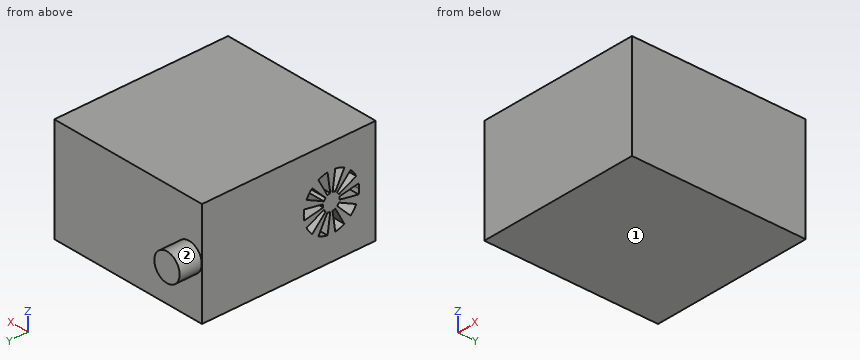
```python
from build123d import *

# Parameters (mm, degrees)
SKETCH1_W           = 73
SKETCH1_H           = 47
BOSS_EXTRUDE1_DEPTH = 78.5
SKETCH2_R           = 6.25
BOSS_EXTRUDE2_DEPTH = 10
CUT_EXTRUDE1_DEPTH  = 10


with BuildPart() as part:
    # Sketch1 → Boss-Extrude1 (new body)
    with BuildSketch(Plane(origin=(0, 0, 0), x_dir=(1, 0, 0), z_dir=(0, 1, 0))):
        with Locations((36.5, 23.5)):
            Rectangle(SKETCH1_W, SKETCH1_H)
    extrude(amount=BOSS_EXTRUDE1_DEPTH)

    # Sketch2 → Boss-Extrude2 (add)
    with BuildSketch(Plane(origin=(0, 78.5, 0), x_dir=(1, 0, 0), z_dir=(0, 1, 0))):
        with Locations(Location((6.35, 23.5, 0), (0, 0, 90))):
            Circle(SKETCH2_R)
    extrude(amount=BOSS_EXTRUDE2_DEPTH)

    # Sketch3 → Cut-Extrude1 (cut)
    with BuildSketch(Plane.ZY):
        with BuildLine():
            ThreePointArc((-21.329397779, 32.310096913), (-22.410553216, 32.452433726), (-23.5, 32.5))
            Line((-23.5, 32.5), (-23.5, 23.75))
            ThreePointArc((-23.5, 23.75), (-23.173165965, 23.735730118), (-22.848819334, 23.693029074))
            Line((-22.848819334, 23.693029074), (-21.329397779, 32.310096913))
        make_face()
        with BuildLine():
            Line((-23.5, 23.75), (-23.5, 32.5))
            ThreePointArc((-23.5, 32.5), (-24.589446784, 32.452433726), (-25.670602221, 32.310096913))
            Line((-25.670602221, 32.310096913), (-24.151180666, 23.693029074))
            ThreePointArc((-24.151180666, 23.693029074), (-23.826834035, 23.735730118), (-23.5, 23.75))
        make_face()
        with BuildLine():
            Line((-18.020360665, 31.234925579), (-21.8561082, 23.370477674))
            ThreePointArc((-21.8561082, 23.370477674), (-21.295805304, 23.033813729), (-20.802475749, 22.604968889))
            Line((-20.802475749, 22.604968889), (-14.508252496, 28.683229631))
            ThreePointArc((-14.508252496, 28.683229631), (-16.152684346, 30.11271243), (-18.020360665, 31.234925579))
        make_face()
        with BuildLine():
            Line((-12.463155089, 25.868394535), (-20.188946527, 21.76051836))
            ThreePointArc((-20.188946527, 21.76051836), (-19.933538064, 21.158813729), (-19.786494742, 20.521899129))
            Line((-19.786494742, 20.521899129), (-11.121649141, 21.739663762))
            ThreePointArc((-11.121649141, 21.739663762), (-11.611793546, 23.86271243), (-12.463155089, 25.868394535))
        make_face()
        with BuildLine():
            Line((-11.121649141, 18.260336238), (-19.786494742, 19.478100871))
            ThreePointArc((-19.786494742, 19.478100871), (-19.933538064, 18.841186271), (-20.188946527, 18.23948164))
            Line((-20.188946527, 18.23948164), (-12.463155089, 14.131605465))
            ThreePointArc((-12.463155089, 14.131605465), (-11.611793546, 16.13728757), (-11.121649141, 18.260336238))
        make_face()
        with BuildLine():
            Line((-21.8561082, 16.629522326), (-18.020360665, 8.765074421))
            ThreePointArc((-18.020360665, 8.765074421), (-16.152684346, 9.88728757), (-14.508252496, 11.316770369))
            Line((-14.508252496, 11.316770369), (-20.802475749, 17.395031111))
            ThreePointArc((-20.802475749, 17.395031111), (-21.295805304, 16.966186271), (-21.8561082, 16.629522326))
        make_face()
        with BuildLine():
            Line((-23.5, 16.25), (-23.5, 7.5))
            ThreePointArc((-23.5, 7.5), (-22.410553216, 7.547566274), (-21.329397779, 7.689903087))
            Line((-21.329397779, 7.689903087), (-22.848819334, 16.306970926))
            ThreePointArc((-22.848819334, 16.306970926), (-23.173165965, 16.264269882), (-23.5, 16.25))
        make_face()
        with BuildLine():
            ThreePointArc((-25.670602221, 7.689903087), (-24.589446784, 7.547566274), (-23.5, 7.5))
            Line((-23.5, 7.5), (-23.5, 16.25))
            ThreePointArc((-23.5, 16.25), (-23.826834035, 16.264269882), (-24.151180666, 16.306970926))
            Line((-24.151180666, 16.306970926), (-25.670602221, 7.689903087))
        make_face()
        with BuildLine():
            ThreePointArc((-32.491747504, 11.316770369), (-30.847315654, 9.88728757), (-28.979639335, 8.765074421))
            Line((-28.979639335, 8.765074421), (-25.1438918, 16.629522326))
            ThreePointArc((-25.1438918, 16.629522326), (-25.704194696, 16.966186271), (-26.197524251, 17.395031111))
            Line((-26.197524251, 17.395031111), (-32.491747504, 11.316770369))
        make_face()
        with BuildLine():
            Line((-34.536844911, 14.131605465), (-26.811053473, 18.23948164))
            ThreePointArc((-26.811053473, 18.23948164), (-27.066461936, 18.841186271), (-27.213505258, 19.478100871))
            Line((-27.213505258, 19.478100871), (-35.878350859, 18.260336238))
            ThreePointArc((-35.878350859, 18.260336238), (-35.388206454, 16.13728757), (-34.536844911, 14.131605465))
        make_face()
        with BuildLine():
            Line((-35.878350859, 21.739663762), (-27.213505258, 20.521899129))
            ThreePointArc((-27.213505258, 20.521899129), (-27.066461936, 21.158813729), (-26.811053473, 21.76051836))
            Line((-26.811053473, 21.76051836), (-34.536844911, 25.868394535))
            ThreePointArc((-34.536844911, 25.868394535), (-35.388206454, 23.86271243), (-35.878350859, 21.739663762))
        make_face()
        with BuildLine():
            Line((-32.491747504, 28.683229631), (-26.197524251, 22.604968889))
            ThreePointArc((-26.197524251, 22.604968889), (-25.704194696, 23.033813729), (-25.1438918, 23.370477674))
            Line((-25.1438918, 23.370477674), (-28.979639335, 31.234925579))
            ThreePointArc((-28.979639335, 31.234925579), (-30.847315654, 30.11271243), (-32.491747504, 28.683229631))
        make_face()
    extrude(amount=-CUT_EXTRUDE1_DEPTH, mode=Mode.SUBTRACT)


solid = part.part
```
Geometry: final body of the model. Coordinates: model frame, mm. Face numbers are marked on the shaded views. A direction names the side the tool comes from. Give positions to 0.01 mm unless a question says otherwise; leave off trailing zeros. Loops run counter-clockwise (first coordinate to the right, second up) from the corner with the lowest first, then second, coordinate; pieces in that order, holes last. Notation, with made-up numbers: (60.5, 38.25) - (86.5, 38.25) arc R38 cw to (86.5, 77.25) - close; hole circle Ø10 at (20.5, 76.25). An arc over 180 degrees is marked (long way). Answer as CSV lines item,"result". Start each with the question number.
(1) Section query A-A (x = 6.35). Give the number of separate pieces and of enclosed holes in the cut face, and give its area (3 significant figures).
(2) Reachability of the marked faces 1 and 2 from +Z, -Z, +X, -X, +Y, -Y: full face, straight path, thin tool, end or side. Return the list, or none.
(3) Pin query (flat end, axial travel): P1, Ø10, axis at x = 11, z = -6, coming from the +Y side; P2, Ø2, axis at y = 28.5, z = -29.5, coming from the -X side. Return the tip coordinate at first contact, or that it passes through.
(4) Section query B-B (x = 39.5). Output: boundary loops of the cut face in (y, z).
(5) Section query C-C (y = 81). Output: boundary loops of the cut face in (x, z).
(6) Section query D-D (z = -31). Output: boundary loops of the cut face in (x, y).
(7) Ray query, line 1 along Y through (x, z) = (57, -22); line 2 along X through (y, z) = (12, -15.5). Return the intervals inside material, ascending. Write a range as [from, to].
Worked answers:
1,separate pieces,"1"
1,enclosed holes,"10"
1,area,"3,570 mm^2"
2,face 1,"-Z, +X, -X, +Y, -Y"
2,face 2,"+Y"
3,P1,"stops at y = 78.5"
3,P2,"stops at x = 10"
4,outline,"(0, -47) - (78.5, -47) - (78.5, 0) - (0, 0) - close"
5,outline,"circle Ø12.5 at (6.35, -23.5)"
6,outline,"(0, 0) - (73, 0) - (73, 78.5) - (0, 78.5) - (0, 30) - (10, 30) - (10, 27.24) - (0, 27.24) - (0, 23.99) - (10, 23.99) - (10, 21.05) - (0, 21.05) - (0, 18.95) - (10, 18.95) - (10, 16.01) - (0, 16.01) - (0, 12.76) - (10, 12.76) - (10, 10) - (0, 10) - close"
7,line 1,"y = [0, 78.5]"
7,line 2,"x = [10, 73]"
